Design review of the part built by this model. Coordinates are the model's own, in mm. Round coordinates to 2 decimals unless told otherwise and drop trailing zeros. Write each loop counter-clockwise with the first axis right and the second up, starting at its lowest first coordinate (ties: lowest second). Pieces come first, ordered by that corner, then holes.
Autodesk Inventor part; units mm, degrees
ref_plane "YZ Plane" through (0, 0, 0) normal (1, 0, 0) x (0, 1, 0)
ref_plane "XZ Plane" through (0, 0, 0) normal (0, 1, 0) x (-1, 0, 0)
ref_plane "XY Plane" through (0, 0, 0) normal (0, 0, 1) x (1, 0, 0)
sketch "Sketch5" plane through (0, 0, 0) normal (1, 0, 0) x (0, 1, 0)
  line L0 (50.6, -39.05) -> (-50.6, -39.05)
  line L1 (-50.6, -39.05) -> (-50.6, 39.05)
  line L2 (-50.6, 39.05) -> (50.6, 39.05)
  line L3 (50.6, 39.05) -> (50.6, -39.05)
  line L4 (50.6, -39.05) -> (-50.6, 39.05) construction
  line L5 (-50.6, -39.05) -> (50.6, 39.05) construction
  point P0 (0, 0)
  dimension "d31" = 78.1
  dimension "d32" = 101.2
extrude "Extrusion2" add sketch "Sketch5" along normal blind 5
sketch "Sketch10" plane through (5, 0, 0) normal (1, 0, 0) x (0, 0, -1)
  line L0 (39.05, 50.6) -> (-39.05, 50.6)
  line L1 (39.05, -50.6) -> (39.05, 50.6)
  point P0 (0, 0)
  point P1 (19.05, 38.1)
  dimension "d93" = 12.5
  dimension "d103" = 20
hole "Hole8" at (5, 38.1, -19.05) direction (-1, 0, 0) diameter 6.8 end through all
sketch "Sketch11" plane through (5, 0, 0) normal (1, 0, 0) x (0, 0, -1)
  circle A0 centre (19.05, 38.1) radius 3.4
  point P0 (0, 0)
  point P1 (-19.05, 38.1)
  dimension "d85" = 38.1
  dimension "d86" = 0
hole "Hole9" at (5, 38.1, 19.05) direction (-1, 0, 0) diameter 6.8 end through all
pattern_linear "Rectangular Pattern1" count 6 spacing 25.4 along (0, -1, 0) of "Hole8"
pattern_linear "Rectangular Pattern2" count 6 spacing 25.4 along (0, -1, 0) of "Hole9"
sketch "Sketch12" plane through (5, 0, 0) normal (1, 0, 0) x (0, 0, -1)
  line L0 (39.05, -50.6) -> (39.05, 50.6)
  line L1 (-39.05, -50.6) -> (39.05, -50.6)
  point P0 (0, 0)
  point P1 (0.04, 0)
  dimension "d101" = 39.01
  dimension "d102" = 50.6
hole "Hole10" at (5, 0, -0.04) direction (-1, 0, 0) diameter 6.75 end through all
properties part number "base_plate"
1) Add section B-B on z = 19.05. State the section outline as (x, y) points, and give its area (3 significant figures).
2) Add section C-C on y = 0. State the section outline as (x, z) points (3 decimals), and give its area (3 significant figures).
3) Add section D-D on y = -12.7. State the section outline as (x, z) points.
4) The part is to be moulded in two halves that separate along Y. For faces 1 (the face through (2.465, 3.295, 0.692)), 2 (the face through (2, -1, 39.05)), 3 (the face through (2.5, 11.7, 15.8)), 4 (the face through (2, -50.6, -1)), say which applies: pulls with the +Y half, pulls with the -Y half, needs draft (parallel to the pull), parting line crosses it, or undercut.
5) For line 1 along Y through (x, z) = (2.05, -19.05); line 2 along Z through (x, y) = (3.95, 38.1); line 3 along Z through (x, y) = (1.15, 0) (3 decimals), list the stretches that pass through material, from the lowest coordinate up.
6) Add section A-A on x = 3.4. Count the separate pieces of the cut face and the enclosed holes in it, and give its area (3 significant figures).
Computed:
1. outline: (0, -50.6) - (5, -50.6) - (5, -41.5) - (0, -41.5) - close; (0, -34.7) - (5, -34.7) - (5, -16.1) - (0, -16.1) - close; (0, -9.3) - (5, -9.3) - (5, 9.3) - (0, 9.3) - close; (0, 16.1) - (5, 16.1) - (5, 34.7) - (0, 34.7) - close; (0, 41.5) - (5, 41.5) - (5, 50.6) - (0, 50.6) - close
1. area: 370 mm2
2. outline: (0, -39.05) - (5, -39.05) - (5, -3.415) - (0, -3.415) - close; (0, 3.335) - (5, 3.335) - (5, 39.05) - (0, 39.05) - close
2. area: 357 mm2
3. outline: (0, -39.05) - (5, -39.05) - (5, -22.45) - (0, -22.45) - close; (0, -15.65) - (5, -15.65) - (5, 15.65) - (0, 15.65) - close; (0, 22.45) - (5, 22.45) - (5, 39.05) - (0, 39.05) - close
4. face 1: undercut
4. face 2: needs draft
4. face 3: undercut
4. face 4: pulls with the -Y half
5. line 1: y = -50.6 to -41.5, -34.7 to -16.1, -9.3 to 9.3, 16.1 to 34.7, 41.5 to 50.6
5. line 2: z = -39.05 to -22.45, -15.65 to 15.65, 22.45 to 39.05
5. line 3: z = -39.05 to -3.415, 3.335 to 39.05
6. separate pieces: 1
6. enclosed holes: 9
6. area: 7,580 mm2
